Model file for the job. Use its own axes, mm. Face numbers are marked on the shaded views. A direction names the side the tool comes from. Coordinates: 2 decimals unless noted, no trailing zeros. Loops run counter-clockwise (first coordinate to the right, second up) from the corner with the lowest first, then second, coordinate; pieces in that order, holes last. Notation, with made-up numbers: (79, 3.25) -> (101, 3.25) arc R10 ccw to (101, 18.25) -> close; hole circle Ø1 at (41, 22). An arc over 180 degrees is marked (long way). Use one line per item in the form item = value.
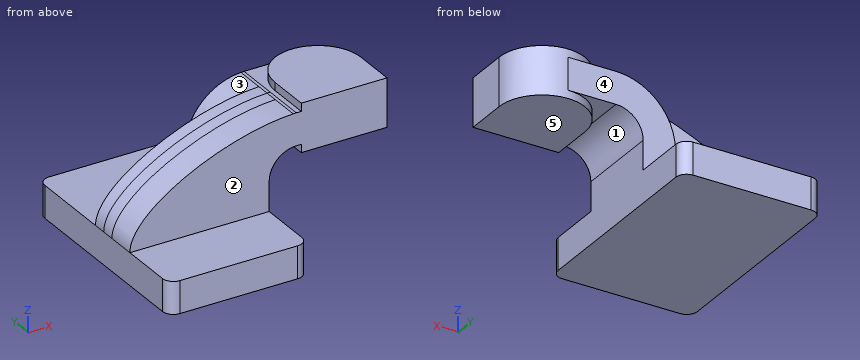
```python
from build123d import *

# Parameters (mm, degrees)
F1_DEPTH = 63.5
F0_W     = 25.4
F0_H     = 19.05
F2_DEPTH = 25.4
F3_DEPTH = 7.9375
F5_R     = 6.35
F0_H_2   = 4.7752
F0_H_3   = 4.7498
F6_DEPTH = 25.4


with BuildPart() as f1:
    # F0 (on Front) → F1 (new body, symmetric)
    with BuildSketch(Plane.XZ):
        Polygon((-41.275, -9.525), (41.275, -9.525), (41.275, 9.525), (22.225, 9.525), (-41.275, 9.525), align=None)
    extrude(amount=F1_DEPTH, both=True)

    # F0 (on Front) → F2 (join, symmetric)
    with BuildSketch(Plane.XZ):
        with BuildLine():
            Line((22.225, 9.525), (41.275, 9.525))
            Line((41.275, 9.525), (41.275, 26.7462))
            ThreePointArc((41.275, 26.7462), (45.9990747262, 38.1511252738), (57.404, 42.8752))
            Line((57.404, 42.8752), (60.325, 42.8752))
            Line((60.325, 42.8752), (60.325, 61.9252))
            Line((60.325, 61.9252), (57.404, 61.9252))
            add(Edge.make_bspline(
                [(55.5422575952, 61.875901909), (56.1662788609, 61.89841175), (56.7869415526, 61.914880349), (57.404, 61.9252)],
                knots=[110.0591294768, 110.0591294768, 110.0591294768, 110.0591294768, 111.7288056011, 111.7288056011, 111.7288056011, 111.7288056011], degree=3))
            ThreePointArc((55.5422575952, 61.875901909), (31.8789507634, 50.9543371128), (22.225, 26.7462))
            Line((22.225, 26.7462), (22.225, 9.525))
        make_face()
        with Locations((73.025, 52.4002)):
            Rectangle(F0_W, F0_H)
    extrude(amount=F2_DEPTH, both=True)

    # F0 (on Front) → F3 (join, symmetric)
    with BuildSketch(Plane.XZ):
        with BuildLine():
            add(Edge.make_bspline(
                [(-41.275, 9.525), (-41.317213665, 32.6592953767), (14.4089885277, 60.3921330151), (55.5422575952, 61.875901909)],
                knots=[0, 0, 0, 0, 110.0591294768, 110.0591294768, 110.0591294768, 110.0591294768], degree=3))
            Line((-41.275, 9.525), (22.225, 9.525))
            Line((22.225, 9.525), (22.225, 26.7462))
            ThreePointArc((22.225, 26.7462), (31.8789507634, 50.9543371128), (55.5422575952, 61.875901909))
        make_face()
    extrude(amount=F3_DEPTH, both=True)

    # F0 (on Front) → F4 (revolve)
    with BuildSketch(Plane.XZ):
        Polygon((85.725, 61.9252), (85.725, 42.8752), (85.725, 38.1), (111.125, 38.1), (111.125, 66.675), (85.725, 66.675), align=None)
    revolve(axis=Axis((85.725, 0, 52.3875), (0, 0, -1)))

    # F5
    f5_edges = [f1.edges().sort_by_distance(p)[0] for p in [
        (-41.275, -63.5, 0),
        (41.275, -63.5, 0),
        (-41.275, 63.5, 0),
        (41.275, 63.5, 0),
    ]]
    fillet(f5_edges, radius=F5_R)

    # F0 (on Front) → F6 (join)
    with BuildSketch(Plane.XZ):
        Polygon((-41.275, -9.525), (41.275, -9.525), (41.275, 9.525), (22.225, 9.525), (-41.275, 9.525), align=None)
        with BuildLine():
            Line((22.225, 9.525), (41.275, 9.525))
            Line((41.275, 9.525), (41.275, 26.7462))
            ThreePointArc((41.275, 26.7462), (45.9990747262, 38.1511252738), (57.404, 42.8752))
            Line((57.404, 42.8752), (60.325, 42.8752))
            Line((60.325, 42.8752), (60.325, 61.9252))
            Line((60.325, 61.9252), (57.404, 61.9252))
            add(Edge.make_bspline(
                [(55.5422575952, 61.875901909), (56.1662788609, 61.89841175), (56.7869415526, 61.914880349), (57.404, 61.9252)],
                knots=[110.0591294768, 110.0591294768, 110.0591294768, 110.0591294768, 111.7288056011, 111.7288056011, 111.7288056011, 111.7288056011], degree=3))
            ThreePointArc((55.5422575952, 61.875901909), (31.8789507634, 50.9543371128), (22.225, 26.7462))
            Line((22.225, 26.7462), (22.225, 9.525))
        make_face()
        with BuildLine():
            add(Edge.make_bspline(
                [(-41.275, 9.525), (-41.317213665, 32.6592953767), (14.4089885277, 60.3921330151), (55.5422575952, 61.875901909)],
                knots=[0, 0, 0, 0, 110.0591294768, 110.0591294768, 110.0591294768, 110.0591294768], degree=3))
            Line((-41.275, 9.525), (22.225, 9.525))
            Line((22.225, 9.525), (22.225, 26.7462))
            ThreePointArc((22.225, 26.7462), (31.8789507634, 50.9543371128), (55.5422575952, 61.875901909))
        make_face()
        with Locations((73.025, 40.4876)):
            Rectangle(F0_W, F0_H_2)
        with Locations((73.025, 52.4002)):
            Rectangle(F0_W, F0_H)
        with Locations((73.025, 64.3001)):
            Rectangle(F0_W, F0_H_3)
        Polygon((85.725, 61.9252), (85.725, 42.8752), (85.725, 38.1), (111.125, 38.1), (111.125, 66.675), (85.725, 66.675), align=None)
    extrude(amount=F6_DEPTH)


solid = f1.part
```
Q1. Band-saw the part on C-C, the plane x = 64. Write the cut outline in (y, z) (3 decimals), and give its area (3 significant figures).
Result:
outline = (-25.4, 38.1) -> (13.16, 38.1) -> (13.16, 42.875) -> (25.4, 42.875) -> (25.4, 61.925) -> (13.16, 61.925) -> (13.16, 66.675) -> (-25.4, 66.675) -> close
area = 1,340 mm2
Q2. Pin check, flat tips, straight feed: pin 1 Ø2.5 at (y, z) = (-15.5, 64.5) entering from -X (3 decimals); pin 2 Ø15.5 at (x, z) = (19, 26.5) entering from +Y; pin 3 Ø6 at (x, y) = (27.5, -34.5) entering from +Z (3 decimals); pin 4 Ø1 at (x, z) = (74, 36.5) entering from +Y. Stop position of each tip, or through.
Result:
pin_1 = 60.325
pin_2 = 25.4
pin_3 = 9.525
pin_4 = through
Q3. Band-saw the part on B-B, the plane y = 43.5. Write the cut outline in (x, z) (3 decimals).
Result:
outline = (-41.275, -9.525) -> (41.275, -9.525) -> (41.275, 9.525) -> (-41.275, 9.525) -> close
Q4. Which spindle directions (+Z, -Z, +X, -X, +Y, -Y) get a long thin tool onto all of the face, cutting with end or side? Do the marked faces 1, 2, 3, 4 and 5. Say none if no direction does.
Result:
face_1 = -Z, +Y, -Y
face_2 = +Z, +X, -X, -Y
face_3 = +Z, -X, +Y
face_4 = +Z, +X, -X, +Y
face_5 = -Z, +X, +Y, -Y
Q5. Band-saw the part on D-D, the plane x = 100. Write the cut outline in (y, z) (3 decimals), and give its area (3 significant figures).
Result:
outline = (-25.4, 38.1) -> (21.009, 38.1) -> (21.009, 66.675) -> (-25.4, 66.675) -> close
area = 1,330 mm2
Q6. Wall check: line 1 along Y through (x, z) = (41, 51); line 2 along Y through (x, z) = (-10, 29); line 3 along Z through (x, y) = (35.5, -44) (3 decimals). Give the ranges that are in metal, low to high.
Result:
line_1 = -25.4 to 25.4
line_2 = -25.4 to 7.94
line_3 = -9.525 to 9.525
Q7. Band-saw the part on A-A, the plane z = -3. Write the cut outline in (x, y) (3 decimals).
Result:
outline = (-41.275, -57.15) arc R6.35 ccw to (-34.925, -63.5) -> (34.925, -63.5) arc R6.35 ccw to (41.275, -57.15) -> (41.275, 57.15) arc R6.35 ccw to (34.925, 63.5) -> (-34.925, 63.5) arc R6.35 ccw to (-41.275, 57.15) -> close
